from build123d import *

# Parameters (mm, degrees)
F0_R     = 15.24
F1_DEPTH = 76.2
F2_R     = 15.24
F3_DEPTH = 12.7


# Not quite as in the source:
# - the program builds the solid bodies; features that only make, move or delete a surface that nothing else refers to are left out


with BuildPart() as f1:
    # F0 (on Front) → F1 (new body)
    with BuildSketch(Plane.XZ):
        with BuildLine():
            ThreePointArc((-30.7586478548, -14.4772019242), (-27.3878303212, -7.5846439713), (-26.2289766602, 0))
            ThreePointArc((-26.2289766602, 0), (-27.6162300636, 8.2793720106), (-31.6264570452, 15.6543670921))
            ThreePointArc((-31.6264570452, 15.6543670921), (-77.0184488356, -0.7312336534), (-30.7586478548, -14.4772019242))
        make_face()
        with Locations((-51.6289766602, 0)):
            Circle(F0_R, mode=Mode.SUBTRACT)
        with BuildLine():
            ThreePointArc((-31.6264570452, 15.6543670921), (-27.6162300636, 8.2793720106), (-26.2289766602, 0))
            ThreePointArc((-26.2289766602, 0), (-27.3878303212, -7.5846439713), (-30.7586478548, -14.4772019242))
            ThreePointArc((-30.7586478548, -14.4772019242), (-0.6990994055, -10.5436994312), (29.4432734756, -13.7819477124))
            ThreePointArc((29.4432734756, -13.7819477124), (25.4048776906, 1.1438261277), (30.7698211259, 15.6457138385))
            ThreePointArc((30.7698211259, 15.6457138385), (-0.4289690246, 10.9553864554), (-31.6264570452, 15.6543670921))
        make_face()
        with BuildLine():
            ThreePointArc((76.179109931, 0), (59.0532885715, 24.014536594), (30.7698211259, 15.6457138385))
            ThreePointArc((30.7698211259, 15.6457138385), (25.4048776906, 1.1438261277), (29.4432734756, -13.7819477124))
            ThreePointArc((29.4432734756, -13.7819477124), (57.9634593807, -24.3627815116), (76.179109931, 0))
        make_face()
        with Locations((50.779109931, 0)):
            Circle(F0_R, mode=Mode.SUBTRACT)
    extrude(amount=F1_DEPTH)

    # F2 (on Front) → F3 (join)
    with BuildSketch(Plane.XZ):
        with Locations((-51.3377061976, 0)):
            Circle(F2_R)
        with Locations((50.8029804159, 0)):
            Circle(F2_R)
    extrude(amount=F3_DEPTH)


solid = f1.part
CAD build for the part. Positions are in the model's coordinates, mm. A direction names the side the tool comes from. Coordinates: 2 decimals unless noted, no trailing zeros. Loops run counter-clockwise (first coordinate to the right, second up) from the corner with the lowest first, then second, coordinate; pieces in that order, holes last. Notation, with made-up numbers: (9.5, 0.5) - (43.5, 0.5) arc R15 ccw to (43.5, 17.5) - close; hole circle Ø10 at (36.5, 76.25). An arc over 180 degrees is marked (long way). Write item = value, one per line. Start each with the question number.
Q1. Pull direction X, two halves, no side cores. Call faces 1 (the flat face through (-1, 0, 0)), 2 (the cylindrical face through (-66.854, -37.567, 0.67)): pulls with the +X half, pulls with the -X half, needs draft (parallel to the pull), parting line crosses it, or undercut.
Q2. Drill centre lines: L1, parallel to X at y = -61, z = -0.5; L2, parallel to X at y = -28, z = 1; L3, parallel to Z at x = -45.5, y = -28. Where is each one in solid material? Low to high.
Q3. Flat gauge pins, fed straight in: pin 1 Ø24 at (x, z) = (-50.5, 3.5) entering from -Y; pin 2 Ø15 at (x, z) = (50.5, 6) entering from -Y; pin 3 Ø10 at (x, y) = (26.5, -9) entering from -Z; pin 4 Ø4 at (x, y) = (-28.5, -9) entering from +Z. Where does each tip first touch, or does it go through?
Q4. Which spindle directions (+Z, -Z, +X, -X, +Y, -Y) get a long thin tool onto all of the face, cutting with end or side? Do faces 3 (the flat face through (-1, -76.2, 0)), 4 (the flat face through (-52, -12.7, 0)). Say none if no direction does.
Q5. Cut at C-C, the plane x = -43. List the corners of the cut face in (y, z).
Q6. Cut at A-A, the plane z = -3. List the corners of the cut face in (x, y), then the cut area to 3 significant figures.
Q7. Cut at B-B, the plane y = -70. List the corners of the cut face in (x, z), then the cut area to 3 significant figures.
Q8. Cut at D-D, the plane z = 5. List the corners of the cut face in (x, y), then the cut area to 3 significant figures.
Computed:
q1.face_1 = needs draft
q1.face_2 = undercut
q2.L1 = -77.02 to -66.86, -36.4 to 35.55, 66.01 to 76.17
q2.L2 = -77.01 to -66.84, -36.42 to 35.57, 65.99 to 76.16
q2.L3 = -24.65 to -13.95, 13.95 to 24.65
q3.pin_1 = -76.2
q3.pin_2 = -12.7
q3.pin_3 = -16.54
q3.pin_4 = 15.31
q4.face_3 = +Z, -Z, +X, -X, -Y
q4.face_4 = -Y
q5.outline = (-76.2, -23.89) - (0, -23.89) - (0, 23.89) - (-76.2, 23.89) - (-76.2, 12.56) - (-12.7, 12.56) - (-12.7, -12.56) - (-76.2, -12.56) - close
q6.outline = (-76.85, -76.2) - (-66.57, -76.2) - (-66.57, 0) - (-76.85, 0) - close; (-66.28, -12.7) - (-36.69, -12.7) - (-36.69, -76.2) - (35.84, -76.2) - (35.84, 0) - (-66.28, 0) - close; (35.86, -12.7) - (65.72, -12.7) - (65.72, -76.2) - (76, -76.2) - (76, 0) - (35.86, 0) - close
q6.area = 7,850 mm²
q7.outline = (-31.63, 15.65) arc R25.4 ccw (long way) to (-30.76, -14.48) arc R128.14 cw to (29.44, -13.78) arc R25.4 ccw (long way) to (30.77, 15.65) arc R106.01 cw to start; hole circle Ø30.48 at (-51.63, 0); hole circle Ø30.48 at (50.78, 0)
q7.area = 3,880 mm²
q8.outline = (-76.53, -76.2) - (-66.03, -76.2) - (-66.03, 0) - (-76.53, 0) - close; (-65.73, -12.7) - (-37.23, -12.7) - (-37.23, -76.2) - (36.38, -76.2) - (36.38, 0) - (-65.73, 0) - close; (36.41, -12.7) - (65.18, -12.7) - (65.18, -76.2) - (75.68, -76.2) - (75.68, 0) - (36.41, 0) - close
q8.area = 7,940 mm²
